Geometry check sheet. Reference: the model listing, model coordinates, mm. Face numbers are marked on the shaded views. A direction names the side the tool comes from. Give positions to 0.01 mm unless a question says otherwise; leave off trailing zeros. Loops run counter-clockwise (first coordinate to the right, second up) from the corner with the lowest first, then second, coordinate; pieces in that order, holes last.
1. Cross-section at A-A, the plane z = -0.5. Record the cut outline in (x, y) (3 decimals).
2. Tool access check on the marked faces 5, 6 and 7. Record the directions out of +Z, -Z, +X, -X, +Y, -Y that give a thin tool (end or side, any length) a straight path to the whole face; none if there is none.
3. Cross-section at B-B, the plane y = 29. Record the cut outline in (x, z) (3 decimals).
4. Release check for a two-part mould opening along X. For the marked faces 1, 2, 3 and 4 record: +X half, -X half, draft (parallel to the pull), parting line (faces both ways), or undercut.
5. Go/stop test with flat-tipped pins: pin 1 Ø1.5 at (x, y) = (86, -20) entering from -Z; pin 2 Ø21.5 at (x, y) = (68.5, 11) entering from +Z; pin 3 Ø1 at (x, z) = (-1.5, 23) entering from -Y; pin 4 Ø8 at (y, z) = (30, 48.5) entering from -X. Record where each tip stops, or that it passes through.
6. Material ranges on L1, parallel to Y at x = 4.5, z = 15; L2, parallel to Z at x = -26.5, y = 38 (3 decimals); L3, parallel to Y at x = 26, z = 30.5, recorded low to high.
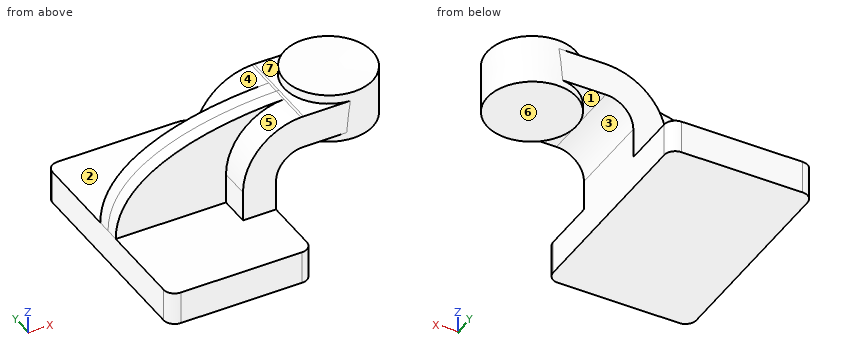
from build123d import *

# Parameters (mm, degrees)
F1_DEPTH = 63.5
F2_DEPTH = 25.4
F3_DEPTH = 7.9375
F5_R     = 6.35


with BuildPart() as f1:
    # F0 (on Front) → F1 (new body, symmetric)
    with BuildSketch(Plane.XZ):
        Polygon((-41.275, 9.525), (-41.275, -9.525), (41.275, -9.525), (41.275, 9.525), (22.225, 9.525), align=None)
    extrude(amount=F1_DEPTH, both=True)

    # F0 (on Front) → F2 (join, symmetric)
    with BuildSketch(Plane.XZ):
        Polygon((85.6770387978, 61.9252), (60.325, 61.9252), (60.325, 42.8752), (85.4846810352, 42.8752), align=None)
        with BuildLine():
            Line((22.225, 9.525), (41.275, 9.525))
            Line((41.275, 9.525), (41.275, 27.0002))
            ThreePointArc((41.275, 27.0002), (45.9246798487, 38.2255201513), (57.15, 42.8752))
            Line((57.15, 42.8752), (60.325, 42.8752))
            Line((60.325, 42.8752), (60.325, 61.9252))
            Line((60.325, 61.9252), (57.15, 61.9252))
            add(Edge.make_bspline(
                [(55.6490044481, 61.8929304371), (56.1503761632, 61.905209471), (56.6507368417, 61.9159599142), (57.15, 61.9252)],
                knots=[110.2646487764, 110.2646487764, 110.2646487764, 110.2646487764, 111.5045361635, 111.5045361635, 111.5045361635, 111.5045361635], degree=3))
            ThreePointArc((55.6490044481, 61.8929304371), (31.9291961404, 51.1593944749), (22.225, 27.0002))
            Line((22.225, 27.0002), (22.225, 9.525))
        make_face()
    extrude(amount=F2_DEPTH, both=True)

    # F0 (on Front) → F3 (join, symmetric)
    with BuildSketch(Plane.XZ):
        with BuildLine():
            add(Edge.make_bspline(
                [(-41.275, 9.525), (-41.522193166, 47.6197025146), (11.061426055, 60.8009414524), (55.6490044481, 61.8929304371)],
                knots=[0, 0, 0, 0, 110.2646487764, 110.2646487764, 110.2646487764, 110.2646487764], degree=3))
            Line((-41.275, 9.525), (22.225, 9.525))
            Line((22.225, 9.525), (22.225, 27.0002))
            ThreePointArc((22.225, 27.0002), (31.9291961404, 51.1593944749), (55.6490044481, 61.8929304371))
        make_face()
    extrude(amount=F3_DEPTH, both=True)

    # F0 (on Front) → F4 (revolve)
    with BuildSketch(Plane.XZ):
        Polygon((85.725, 66.675), (85.6770387978, 61.9252), (85.4846810352, 42.8752), (85.436463356, 38.1), (111.125, 38.1), (111.125, 66.675), align=None)
    revolve(axis=Axis((85.580731678, 0, 52.3875), (-0.0100970056, 0, -0.9999490239)))

    # F5
    f5_edges = [f1.edges().sort_by_distance(p)[0] for p in [
        (-41.275, -63.5, 0),
        (41.275, -63.5, 0),
        (41.275, 63.5, 0),
        (-41.275, 63.5, 0),
    ]]
    fillet(f5_edges, radius=F5_R)


solid = f1.part
Result:
1. outline: (-41.275, -57.15) arc R6.35 ccw to (-34.925, -63.5) - (34.925, -63.5) arc R6.35 ccw to (41.275, -57.15) - (41.275, 57.15) arc R6.35 ccw to (34.925, 63.5) - (-34.925, 63.5) arc R6.35 ccw to (-41.275, 57.15) - close
2. face 5: +Z, -X, -Y
2. face 6: -Z
2. face 7: +Z, -X
3. outline: (-41.275, -9.525) - (41.275, -9.525) - (41.275, 9.525) - (-41.275, 9.525) - close
4. face 1: undercut
4. face 2: draft
4. face 3: undercut
4. face 4: -X half
5. pin 1: stops at z = 38.29
5. pin 2: stops at z = 67.19
5. pin 3: stops at y = -7.94
5. pin 4: passes through
6. L1: y = -7.94 to 7.94
6. L2: z = -9.525 to 9.525
6. L3: y = -25.4 to 25.4
